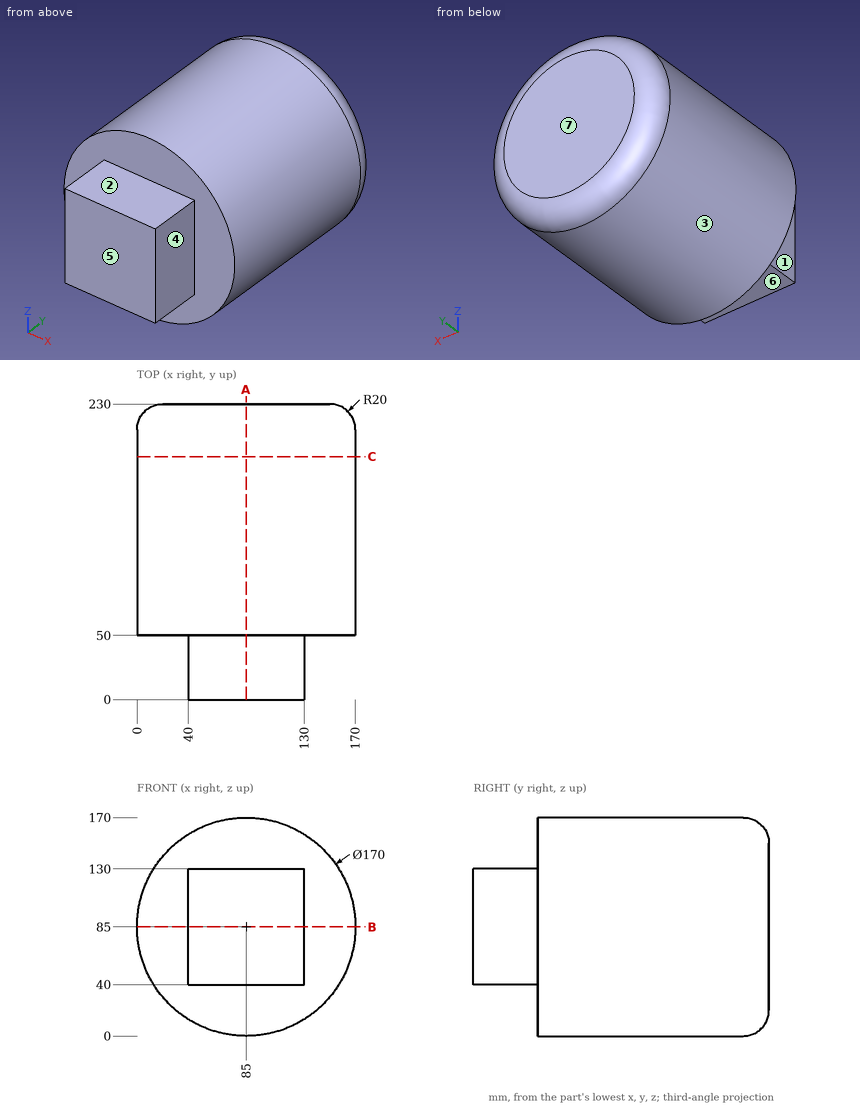
Verification items for this drawing (mm, ordinates from the low corner). A direction names the side the tool comes from. Give positions to 0.01 mm unless a question says otherwise; leave off trailing zeros. Write each loop counter-clockwise with the first axis right and the second up, starting at its lowest first coordinate (ties: lowest second). Pieces come first, ordered by that corner, then holes. Notation, with made-up numbers: (15, 2.5) - (67, 2.5) arc R10 ccw to (67, 21.5) - close; hole circle Ø3 at (67, 38.25). An arc over 180 degrees is marked (long way). Answer as CSV lines item,"result". Start each with the question number.
1. Depth check by flat-ended pin: pin 1 (3 mm diameter, centred on x = 37, y = 84.5, fed in from +Z); pin 2 (4 mm diameter, centred on x = 148.5, z = 114.5, fed in from +Y); pin 3 (25 mm diameter, centred on x = 87.5, y = 32.5, fed in from -Z); pin 4 (12 mm diameter, centred on x = 41, z = 34.5, fed in from +Y). Enter the tip coordinate at first touch or a pass-through.
2. Draft check along Y on the marked faces 5, 6 and 7. Enter one of: pulls with the +Y half, pulls with the -Y half, needs draft (parallel to the pull), parting line crosses it, or undercut.
3. Sectioned sample at A-A (x = 85). Record the boundary of the cut face in (y, z), then the cut area to 3 significant figures.
4. Thickness scan on line 1 (Y direction, x = 137.5, z = 114); line 2 (Y direction, x = 150, z = 71); line 3 (Z direction, x = 115, y = 21.5). Record the ranges inside material, lowest first.
5. Set-up check for the marked faces 1, 2, 3 and 4: record each of +Z, -Z, +X, -X, +Y, -Y from which the full face is reachable in a straight line by a thin tool's end or side.
6. Sectioned sample at C-C (y = 189). Record the boundary of the cut face in (x, z).
7. Sectioned sample at B-B (z = 85). Record the boundary of the cut face in (x, y), then the cut area to 3 significant figures.
Derived:
1,pin 1,"z = 156.15"
1,pin 2,"y = 229.77"
1,pin 3,"z = 40"
1,pin 4,"y = 230"
2,face 5,"pulls with the -Y half"
2,face 6,"needs draft"
2,face 7,"pulls with the +Y half"
3,outline,"(0, 40) - (50, 40) - (50, 0) - (210, 0) arc R20 ccw to (230, 20) - (230, 150) arc R20 ccw to (210, 170) - (50, 170) - (50, 130) - (0, 130) - close"
3,area,"34,900 mm²"
4,line 1,"50 to 230"
4,line 2,"50 to 229.94"
4,line 3,"40 to 130"
5,face 1,"+Z, -Z, -X, -Y"
5,face 2,"+Z, +X, -X, -Y"
5,face 3,"+Y, -Y"
5,face 4,"+Z, -Z, +X, -Y"
6,outline,"circle Ø170 at (85, 85)"
7,outline,"(0, 50) - (40, 50) - (40, 0) - (130, 0) - (130, 50) - (170, 50) - (170, 210) arc R20 ccw to (150, 230) - (20, 230) arc R20 ccw to (0, 210) - close"
7,area,"34,900 mm²"
